```python
from build123d import *

# Parameters (mm, degrees)
SKETCH3_R           = 125
BOSS_EXTRUDE1_DEPTH = 35
SKETCH4_R           = 120
CUT_EXTRUDE1_DEPTH  = 65
SKETCH5_R           = 7.5
CUT_EXTRUDE2_DEPTH  = 189.348082018


with BuildPart() as part:
    # Sketch3 → Boss-Extrude1 (new, symmetric)
    with BuildSketch(Plane(origin=(0, 0, 0), x_dir=(1, 0, 0), z_dir=(0, 1, 0))):
        with Locations(Location((0, 0, 0), (0, 0, 270))):
            Circle(SKETCH3_R)
    extrude(amount=BOSS_EXTRUDE1_DEPTH, both=True)

    # Sketch4 → Cut-Extrude1 (cut)
    with BuildSketch(Plane(origin=(0, 35, 0), x_dir=(1, 0, 0), z_dir=(0, 1, 0))):
        with Locations(Location((0, 0, 0), (0, 0, 270))):
            Circle(SKETCH4_R)
    extrude(amount=-CUT_EXTRUDE1_DEPTH, mode=Mode.SUBTRACT)

    # Sketch5 → Cut-Extrude2 (cut, through all)
    with BuildSketch(Plane(origin=(0, -30, 0), x_dir=(1, 0, 0), z_dir=(0, 1, 0))):
        with Locations(Location((0, 0, 0), (0, 0, 270))):
            Circle(SKETCH5_R)
    extrude(amount=-CUT_EXTRUDE2_DEPTH, mode=Mode.SUBTRACT)


solid = part.part
```
Geometry: final body of the model. Coordinates: model frame, mm. A direction names the side the tool comes from. Coordinates: 2 decimals unless noted, no trailing zeros. Order: outer loops, then holes, each group sorted by start corner. A loop starts at its lowest first (then second) coordinate and runs counter-clockwise, first axis right, second up. Notation, with made-up numbers: (-6, 32) - (5, 32) arc R23 cw to (5, 64) - close; hole circle Ø11 at (-13.5, 6.5). An arc over 180 degrees is marked (long way). Return JSON: item names as keys, results as strings. Group by question number.
1. Pin query (flat end, axial travel): pin 1 (6 mm diameter, centred on x = 79.5, z = -48.5, fed in from +Y); pin 2 (8 mm diameter, centred on y = -7, z = 53, fed in from -X); pin 3 (10 mm diameter, centred on x = -61.5, y = 21, fed in from -Z); pin 4 (13.5 mm diameter, centred on x = 0, z = 0, fed in from -Y). Return the tip coordinate at first contact, or that it passes through.
2. Cut plane D-D (z = 77). Output: boundary loops of the cut face in (x, y), plus the area to 3 significant figures.
3. Set-up query: faces 1 (the face through (112, 35, -47)), 2 (the face through (5.276, 2.955, -119.884)). Return all of +Z, -Z, +X, -X, +Y, -Y with unobstructed straight access to the full face (end or side cutting, diameter ignored); none if empty.
4. Cut plane B-B (z = 0). Output: boundary loops of the cut face in (x, y).
5. Cut plane C-C (y = 12). Output: boundary loops of the cut face in (x, z), plus the area to 3 significant figures.
6. Pull-direction query (Z, two-part tool) for faces 3 (the face through (0.33, -32.465, -7.493)), 4 (the face through (-26, -35, -2)), 5 (the face through (5.5, 0.49, -124.88)); classes: pulls with the +Z half, pulls with the -Z half, needs draft (parallel to the pull), parting line crosses it, or undercut.
7. Cut plane A-A (x = 0). Output: boundary loops of the cut face in (y, z), plus the area to 4 significant figures.
8. Material intervals for line 1 along X through (y, z) = (-33.1, 0); line 2 along X through (y, z) = (2, 0); line 3 along Y through (x, z) = (-74.5, -69), sorted ascending. Write a range as [from, to].
Resolved:
{
 "1": {"pin 1": "stops at y = -30", "pin 2": "stops at x = -115", "pin 3": "stops at z = -111.5", "pin 4": "passes through"},
 "2": {"outline": "(-98.47, -35) - (98.47, -35) - (98.47, 35) - (92.04, 35) - (92.04, -30) - (-92.04, -30) - (-92.04, 35) - (-98.47, 35) - close", "area": "1,820 mm²"},
 "3": {"face 1": "+Z, -Z, +X, -X, +Y", "face 2": "+Y"},
 "4": {"outline": "(-125, -35) - (-7.5, -35) - (-7.5, -30) - (-120, -30) - (-120, 35) - (-125, 35) - close; (7.5, -35) - (125, -35) - (125, 35) - (120, 35) - (120, -30) - (7.5, -30) - close"},
 "5": {"outline": "circle Ø250 at (0, 0); hole circle Ø240 at (0, 0)", "area": "3,850 mm²"},
 "6": {"face 3": "undercut", "face 4": "needs draft", "face 5": "parting line crosses it"},
 "7": {"outline": "(-35, -125) - (35, -125) - (35, -120) - (-30, -120) - (-30, -7.5) - (-35, -7.5) - close; (-35, 7.5) - (-30, 7.5) - (-30, 120) - (35, 120) - (35, 125) - (-35, 125) - close", "area": "1,825 mm²"},
 "8": {"line 1": "x = [-125, -7.5], [7.5, 125]", "line 2": "x = [-125, -120], [120, 125]", "line 3": "y = [-35, -30]"}
}
